```python
from build123d import *

# Parameters (mm, degrees)
SKETCH_1_R      = 6.5
SKETCH_1_R_2    = 2.1
SKETCH_1_R_3    = 1.6
EXTRUDE_2_DEPTH = 4


with BuildPart() as part:
    # 草图1 → 凸台-拉伸2 (new body)
    with BuildSketch(Plane(origin=(0, 0, 0), x_dir=(1, 0, 0), z_dir=(0, 1, 0))):
        with BuildLine():
            Line((-26.580295873, -66.404426064), (-26.580295873, 0))
            ThreePointArc((-26.580295873, 0), (0, 26.580295873), (26.580295873, 0))
            Line((26.580295873, 0), (26.580295873, -66.404426064))
            ThreePointArc((26.580295873, -66.404426064), (25.965220113, -67.889350304), (24.480295873, -68.504426064))
            Line((24.480295873, -68.504426064), (-24.480295873, -68.504426064))
            ThreePointArc((-24.480295873, -68.504426064), (-25.965220113, -67.889350304), (-26.580295873, -66.404426064))
        make_face()
        with Locations(Location((0, 0, 0), (0, 0, 270))):
            Circle(SKETCH_1_R, mode=Mode.SUBTRACT)
        with Locations(Location((0, 20, 0), (0, 0, 270))):
            Circle(SKETCH_1_R_2, mode=Mode.SUBTRACT)
        with Locations(Location((-17.320508076, -10, 0), (0, 0, 270))):
            Circle(SKETCH_1_R_2, mode=Mode.SUBTRACT)
        with Locations(Location((17.32050808, -10, 0), (0, 0, 270))):
            Circle(SKETCH_1_R_2, mode=Mode.SUBTRACT)
        with Locations(Location((21.580295873, -63.504426064, 0), (0, 0, 270))):
            Circle(SKETCH_1_R_3, mode=Mode.SUBTRACT)
        with Locations(Location((13.580295873, -63.504426064, 0), (0, 0, 270))):
            Circle(SKETCH_1_R_3, mode=Mode.SUBTRACT)
        with Locations(Location((-13.580295873, -63.504426064, 0), (0, 0, 90))):
            Circle(SKETCH_1_R_3, mode=Mode.SUBTRACT)
        with Locations(Location((-21.580295873, -63.504426064, 0), (0, 0, 90))):
            Circle(SKETCH_1_R_3, mode=Mode.SUBTRACT)
    extrude(amount=EXTRUDE_2_DEPTH)


solid = part.part
```
Can you work these out from the model? Positions are in its coordinate system, mm. Coordinates: 2 decimals unless noted, no trailing zeros. Loops run counter-clockwise (first coordinate to the right, second up) from the corner with the lowest first, then second, coordinate; pieces in that order, holes last. Notation, with made-up numbers: M 53.5,9.25 L 59.5,9.25 A35 ccw 59.5,42.25 Z; hole C 5.5,48 d2. An arc over 180 degrees is marked long. Put each result on its own line as item: value. Start each with the question number.
(1) We'd pull the mould along X, two halves only. Please class faces 1 (the face through (-22.06, 1.97, 61.98)), 2 (the face through (-0.584, 1.972, -26.574)), 3 (the face through (0, 4, 20)): +X half, -X half, draft (parallel to the pull), parting line (faces both ways), or undercut.
(2) Imagine slicing it at A-A on z = 10. List the corners of the cut face in (x, y) for me, and give its area (3 significant figures).
(3) Imagine slicing it at C-C on z = -4. List the corners of the cut face in (x, y) for me.
(4) Imagine slicing it at B-B on x = 0. List the corners of the cut face in (y, z) for me.
(5) Imagine slicing it at D-D on x = -18.5. List the corners of the cut face in (y, z) for me, and give its area (3 significant figures).
(6) Will this pin go through, and if not, where does the flat tip stop? pin 1 Ø11.5 at (x, z) = (0, 0) entering from +Y.
(7) I need wall thicknesses on probe 1 along X at (y, z) = (2, 10); probe 2 along Z at (x, y) = (-0.5, 0.4); probe 3 along Z at (x, y) = (-1.5, 3.55). Which ranges of each line are inside material? Lowest first, please.
Worked answers:
1. face 1: undercut
1. face 2: parting line
1. face 3: draft
2. outline: M -26.58,0 L -19.42,0 L -19.42,4 L -26.58,4 Z; M -15.22,0 L 15.22,0 L 15.22,4 L -15.22,4 Z; M 19.42,0 L 26.58,0 L 26.58,4 L 19.42,4 Z
2. area: 179 mm2
3. outline: M -26.28,0 L -5.12,0 L -5.12,4 L -26.28,4 Z; M 5.12,0 L 26.28,0 L 26.28,4 L 5.12,4 Z
4. outline: M 0,-26.58 L 4,-26.58 L 4,-22.1 L 0,-22.1 Z; M 0,-17.9 L 4,-17.9 L 4,-6.5 L 0,-6.5 Z; M 0,6.5 L 4,6.5 L 4,68.5 L 0,68.5 Z
5. outline: M 0,-19.09 L 4,-19.09 L 4,8.26 L 0,8.26 Z; M 0,11.74 L 4,11.74 L 4,68.5 L 0,68.5 Z
5. area: 336 mm2
6. pin 1: passes through
7. probe 1: x = -26.58 to -19.42, -15.22 to 15.22, 19.42 to 26.58
7. probe 2: z = -26.58 to -22.04, -17.96 to -6.48, 6.48 to 68.5
7. probe 3: z = -26.54 to -21.47, -18.53 to -6.32, 6.32 to 68.5
